Autodesk Inventor part; units mm, degrees
ref_plane "YZ Plane" through (0, 0, 0) normal (1, 0, 0) x (0, 1, 0)
ref_plane "XZ Plane" through (0, 0, 0) normal (0, 1, 0) x (-1, 0, 0)
ref_plane "XY Plane" through (0, 0, 0) normal (0, 0, 1) x (1, 0, 0)
sketch "Esquisse1" plane through (0, 0, 0) normal (0, 0, 1) x (1, 0, 0)
  line L0 (-5, -2.9) -> (5, -2.9)
  line L1 (5, -2.9) -> (5, 2.9)
  line L2 (5, 2.9) -> (-5, 2.9)
  line L3 (-5, 2.9) -> (-5, -2.9)
  line L4 (-5, -2.9) -> (5, 2.9) construction
  line L5 (5, -2.9) -> (-5, 2.9) construction
  point P0 (0, 0)
  dimension "d0" = 10
  dimension "d1" = 5.8
extrude "Extrusion1" add sketch "Esquisse1" along normal blind 3.5
chamfer "Chanfrein1" distance 2.5 angle 45 2 edges at (5, 0, 0) (-5, 0, 0)
fillet "Congé1" radius 2 2 edges at (5, 2.9, 3) (-5, -2.9, 3)
fillet "Congé2" radius 0.25 12 edges at (0, 2.9, 0) (5, -1, 2.5) (4.4142, 2.3142, 1.9142) (3.75, -2.9, 1.25) (0, -2.9, 0) (2.5, 0, 0) (-2.5, 0, 0) (-3.75, 2.9, 1.25) (-5, 1, 2.5) (-4.4142, -2.3142, 1.9142) (-5, 2.9, 3) (5, -2.9, 3)
sketch "Esquisse2" plane through (0, 0, 3.5) normal (0, 0, 1) x (1, 0, 0)
  line L0 (3, 2.9) -> (-3, 2.9)
  line L1 (-3, 2.9) -> (-3, -2.9)
  line L2 (-3, -2.9) -> (3, -2.9)
  line L3 (3, -2.9) -> (3, 2.9)
  line L4 (3, 2.9) -> (-3, -2.9) construction
  line L5 (-3, 2.9) -> (3, -2.9) construction
  line L6 (-3, -2.9) -> (4.75, -2.9)
  point P0 (0, 0)
  dimension "d9" = 6
extrude "Extrusion2" add sketch "Esquisse2" along normal blind 1
fillet "Congé3" radius 2 2 edges at (3, 2.9, 4) (-3, -2.9, 4)
fillet "Congé4" radius 0.25 2 edges at (-3, 2.9, 4) (3, -2.9, 4)
sketch "Esquisse3" plane through (0, 0, 4.5) normal (0, 0, 1) x (1, 0, 0)
  point P0 (0, 0)
  point P1 (0, 0)
hole "Perçage1" at (0, 0, 4.5) direction (0, 0, -1) diameter 2.459 depth 8.8 tip angle 118
chamfer "Chanfrein2" distance 0.25 angle 45 2 edges at (0, 1.2295, 4.5) (0, 1.2295, 0)
properties part number "Noix M3" material "Acier inoxydable"
Geometry check sheet. Reference: the model listing, model coordinates, mm. A direction names the side the tool comes from. Give positions to 0.01 mm unless a question says otherwise; leave off trailing zeros. Loops run counter-clockwise (first coordinate to the right, second up) from the corner with the lowest first, then second, coordinate; pieces in that order, holes last. Notation, with made-up numbers: M -35,66.5 L 15,66.5 A30 ccw 15,100.5 Z; hole C -3.5,72 d2. An arc over 180 degrees is marked long. Write item = value, one per line. Start each with the question number.
1. Section check B-B, the plane y = 0. Enter the section's corners in (x, z), plus the area to 3 significant figures.
2. Section check A-A, the plane x = 0. Enter the section's corners in (y, z).
3. Thickness scan on probe 1 along X at (y, z) = (0, 2.7); probe 2 along Y at (x, z) = (0, 3.35); probe 3 along X at (y, z) = (-1.05, 2.5). Record the ranges inside material, lowest first.
4. Tool access check on faces 1 (the face through (-4.2, -2.5, 2.8)), 2 (the face through (2.4, 2.33, 3.99)), 3 (the face through (-2.4, -2.33, 3.99)), 4 (the face through (1, -2.9, 2)), 5 (the face through (3, -1, 4)). Record the directions out of +Z, -Z, +X, -X, +Y, -Y that give a thin tool (end or side, any length) a straight path to the whole face; none if there is none.
5. Go/stop test with flat-tipped pins: P1, Ø2, axis at x = 0, y = 0, coming from the -Z side; P2, Ø3, axis at x = 2, y = 0, coming from the -Z side. Record where each tip stops, or that it passes through.
Values follow:
q1.outline = M -5,2.6 A0.25 ccw -4.93,2.43 L -2.57,0.07 A0.25 ccw -2.4,0 L -1.48,0 L -1.23,0.25 L -1.23,4.25 L -1.48,4.5 L -3,4.5 L -3,3.5 L -5,3.5 Z; M 1.23,0.25 L 1.48,0 L 2.4,0 A0.25 ccw 2.57,0.07 L 4.93,2.43 A0.25 ccw 5,2.6 L 5,3.5 L 3,3.5 L 3,4.5 L 1.48,4.5 L 1.23,4.25 Z
q1.area = 23.6 mm^2
q2.outline = M -2.9,0.25 A0.25 ccw -2.65,0 L -1.48,0 L -1.23,0.25 L -1.23,4.25 L -1.48,4.5 L -2.9,4.5 Z; M 1.23,0.25 L 1.48,0 L 2.65,0 A0.25 ccw 2.9,0.25 L 2.9,4.5 L 1.48,4.5 L 1.23,4.25 Z
q3.probe_1 = -5 to -1.23, 1.23 to 5
q3.probe_2 = -2.9 to -1.23, 1.23 to 2.9
q3.probe_3 = -4.97 to -0.64, 0.64 to 4.98
q4.face_1 = +Z, -Z, -X, -Y
q4.face_2 = +Z, +X, +Y
q4.face_3 = +Z, -X, -Y
q4.face_4 = +Z, -Z, +X, -X, -Y
q4.face_5 = +Z, +X, +Y, -Y
q5.P1 = through
q5.P2 = 0
